Build history of the part. All positions in model axes, mm. A direction names the side the tool comes from. Give positions to 0.01 mm unless a question says otherwise; leave off trailing zeros. Order: outer loops, then holes, each group sorted by start corner. A loop starts at its lowest first (then second) coordinate and runs counter-clockwise, first axis right, second up. Notation, with made-up numbers: M 45.25,-15.5 L 87.25,-15.5 A25 ccw 87.25,-0.5 Z; hole C 11,48.25 d9. An arc over 180 degrees is marked long. Answer as CSV lines item,"result".
Autodesk Inventor part; units mm, degrees
ref_plane "YZ Plane" through (0, 0, 0) normal (1, 0, 0) x (0, 1, 0)
ref_plane "XZ Plane" through (0, 0, 0) normal (0, 1, 0) x (-1, 0, 0)
ref_plane "XY Plane" through (0, 0, 0) normal (0, 0, 1) x (1, 0, 0)
sketch "Sketch1" plane through (0, 0, 0) normal (0, 0, 1) x (1, 0, 0)
  circle A0 centre (2.5, 2.5) radius 5
  circle A1 centre (0.5, 5.9641) radius 1
  circle A2 centre (2.5, 2.5) radius 2.5
  point P0 (0, 0)
  point P1 (0, 0)
  point P2 (-2.5, 2.5)
  point P3 (0, 6.8301)
  point P4 (0, -1.8301)
  point P5 (0.5, 6.9641)
  point P6 (0, 2.5)
  point P7 (2.0779, 4.9641)
  dimension "d0" = 5
sketch "Sketch2" plane through (0, 0, 0) normal (0, 0, 1) x (1, 0, 0)
  circle A0 centre (2.5, 2.5) radius 5
  circle A1 centre (0.5, 5.9641) radius 1
  circle A2 centre (2.5, 2.5) radius 2.5
  point P0 (0, 0)
  point P1 (0, 0)
  point P2 (0, 0)
  point P3 (-2.5, 2.5)
  point P4 (0, 6.8301)
  point P5 (0, -1.8301)
  point P6 (0.5, 6.9641)
  point P7 (0, 2.5)
  point P8 (2.0779, 4.9641)
  dimension "d1" = 5
extrude "Extrusion1" add sketch "Sketch1" along normal blind 2 contours A1
extrude "Extrusion2" add sketch "Sketch2" against normal blind 2 contours A1 | A0 | A2
sketch "Sketch3" plane through (2.5, 2.5, 0) normal (0, 0, 1) x (1, 0, 0)
  circle A0 centre (0, 0) radius 5
  circle A1 centre (-2, 3.4641) radius 1
  arc A2 (-2.1651, -1.25) -> (2.1651, 1.25) centre (0, 0) ccw
  circle A3 centre (0, 0) radius 5
  line L0 (0, 0) -> (2.1651, 1.25)
  line L1 (0, 0) -> (-2.1651, -1.25)
  circle A4 centre (-2, 3.4641) radius 1
  point P0 (-2.5, -2.5)
  point P1 (-2.5, -2.5)
  point P2 (-2.5, -2.5)
  point P3 (-2.5, -2.5)
  point P4 (-5, 0)
  point P5 (-2.5, 4.3301)
  point P6 (-2.5, -4.3301)
  point P7 (-2, 4.4641)
  point P8 (-2.5, 0)
  point P9 (-0.4221, 2.4641)
  point P10 (-2.5, 4.3301)
  dimension "d6" = 5
extrude "Extrusion3" add sketch "Sketch3" along normal blind 2 contours L1 L0 A2
sketch "Sketch4" plane through (2.5, 2.5, -2) normal (0, 0, -1) x (-1, 0, 0)
  line L0 (-2.1651, 1.25) -> (2.1651, -1.25)
  circle A0 centre (0, 0) radius 1.5
  point P0 (2.5, -2.5)
  dimension "d9" = 3
extrude "Extrusion4" cut sketch "Sketch4" against normal up to surface (4 mm away)
properties part number "C"
Item 1: Band-saw the part on B-B (y = 2.5). Give the cut face in (x, z), and give its area (3 significant figures).
Geometry says:
outline,"M -2.5,-2 L 1,-2 L 1,0 L -2.5,0 Z; M 4,-2 L 7.5,-2 L 7.5,0 L 5,0 L 5,2 L 4,2 Z"
area,"16.0 mm2"
Item 2: Probe line 1 along Y through (x, z) = (2.5, -0.2); line 2 along Y through (x, z) = (2.5, 0.55). List the from-to ranges inside material, lowest first. Write a range as from..to.
Geometry says:
line 1,"y = -2.5..1, 4..7.5"
line 2,"y = 0..1"
Item 3: 3-axis set-ups, long thin cutter, end or side, ignore diameter. For faces 1 (the flat face through (4, 4, 0)), 2 (the flat face through (0.77, 1.5, 0.99)), 3 (the flat face through (4.238, 3.503, 0.986)): which of +Z, -Z, +X, -X, +Y, -Y reach the whole face in a straight line?
Geometry says:
face 1,"+Z"
face 2,"+Z, -X"
face 3,"+Z, -X, +Y"
Item 4: Band-saw the part on C-C (z = -0.25). Give the cut face in (x, y).
Geometry says:
outline,"C 2.5,2.5 d10; hole C 2.5,2.5 d3"
Item 5: Pull direction X, two halves, no side cores. Call faces 4 (the cylindrical face through (2.825, 1.036, -0.472)), 5 (the flat face through (4, 1, 2)), 6 (the cylindrical face through (0.37, 4.973, 0.986)): released by +X, released by -X, zero draft, split by the parting line, or undercut.
Geometry says:
face 4,"undercut"
face 5,"zero draft"
face 6,"split by the parting line"
Item 6: Band-saw the part on A-A (x = 2.5). Give the cut face in (y, z), and give its area (3 significant figures).
Geometry says:
outline,"M -2.5,-2 L 1,-2 L 1,2 L 0,2 L 0,0 L -2.5,0 Z; M 4,-2 L 7.5,-2 L 7.5,0 L 4,0 Z"
area,"16.0 mm2"
Item 7: Drop flat-ended pins along their axis: pin 1 (1.5 mm diameter, centred on y = 0.5, z = -0.5, fed in from +X); pin 2 (1.8 mm diameter, centred on x = 2.5, y = 2.5, fed in from -Z); pin 3 (1.5 mm diameter, centred on x = 5, z = -1, fed in from +Y); pin 4 (1.5 mm diameter, centred on x = 4.5, z = 1, fed in from -Y). Give the stop position or say it passes through.
Geometry says:
pin 1,"stops at x = 7.34"
pin 2,"passes through"
pin 3,"stops at y = 7.18"
pin 4,"stops at y = 0.33"
Item 8: Band-saw the part on D-D (y = 0.75). Give the cut face in (x, z), and give its area (3 significant figures).
Geometry says:
outline,"M -2.18,-2 L 7.18,-2 L 7.18,0 L 4.29,0 L 4.29,2 L 0.71,2 L 0.71,0 L -2.18,0 Z"
area,"25.9 mm2"
